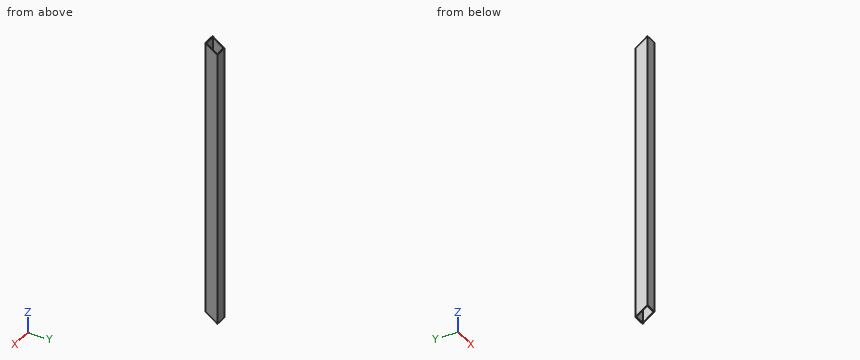
from build123d import *

# Parameters (mm, degrees)
SKETCH1_W           = 50.8
SKETCH1_H           = 50.8
SKETCH1_W_2         = 44.45
SKETCH1_H_2         = 44.45
BOSS_EXTRUDE1_DEPTH = 1231.9
CUT_EXTRUDE1_DEPTH  = 1234.20858333
CUT_EXTRUDE2_DEPTH  = 1234.20858333


with BuildPart() as part:
    # Sketch1 → Boss-Extrude1 (new body)
    with BuildSketch(Plane.XY):
        Rectangle(SKETCH1_W, SKETCH1_H)
        Rectangle(SKETCH1_W_2, SKETCH1_H_2, mode=Mode.SUBTRACT)
    extrude(amount=BOSS_EXTRUDE1_DEPTH)

    # Sketch2 → Cut-Extrude1 (cut, through all)
    with BuildSketch(Plane.ZY.offset(25.4)):
        Polygon((0, 25.4), (36.908360423, -25.4), (0, -25.4), align=None)
    extrude(amount=-CUT_EXTRUDE1_DEPTH, mode=Mode.SUBTRACT)

    # Sketch3 → Cut-Extrude2 (cut, through all)
    with BuildSketch(Plane.ZY.offset(25.4)):
        Polygon((1231.9, -25.4), (1194.991639577, 25.4), (1231.9, 25.4), align=None)
    extrude(amount=-CUT_EXTRUDE2_DEPTH, mode=Mode.SUBTRACT)


solid = part.part
Build history of the part. All positions in model axes, mm. Coordinates: 2 decimals unless noted, no trailing zeros. Write each loop counter-clockwise with the first axis right and the second up, starting at its lowest first coordinate (ties: lowest second). Pieces come first, ordered by that corner, then holes.
(1) Cut at C-C on y = 10. List the corners of the cut face in (x, z) (3 decimals), and give its area (3 significant figures).
(2) Cut at B-B on x = -3. List the corners of the cut face in (y, z) (3 decimals), and give its area (3 significant figures).
(3) Cut at A-A on z = 918.5. List the corners of the cut face in (x, y) (3 decimals), and give its area (3 significant figures).
(4) Pin check, flat tip, straight feed: pin 1 Ø4 at (x, y) = (17, -20) entering from +Z. Stop position of the tip, or through.
(5) Drill centre lines: line 1 (X direction, y = -2, z = 1163) (3 decimals); line 2 (Z direction, x = -10, y = 23). Where is each one in solid material? Low to high.
Working result:
1. outline: (-25.4, 11.189) - (-22.225, 11.189) - (-22.225, 1206.18) - (-25.4, 1206.18) - close; (22.225, 11.189) - (25.4, 11.189) - (25.4, 1206.18) - (22.225, 1206.18) - close
1. area: 7,590 mm2
2. outline: (-25.4, 36.908) - (-22.225, 34.602) - (-22.225, 1229.593) - (-25.4, 1231.9) - close; (22.225, 2.307) - (25.4, 0) - (25.4, 1194.992) - (22.225, 1197.298) - close
2. area: 7,590 mm2
3. outline: (-25.4, -25.4) - (25.4, -25.4) - (25.4, 25.4) - (-25.4, 25.4) - close; hole (-22.225, -22.225) - (22.225, -22.225) - (22.225, 22.225) - (-22.225, 22.225) - close
3. area: 605 mm2
4. pin 1: passes through
5. line 1: x = -25.4 to -22.225, 22.225 to 25.4
5. line 2: z = 1.74 to 1196.74
